Verification items for the finished model (mm, model axes). A direction names the side the tool comes from. Coordinates: 2 decimals unless noted, no trailing zeros. Loops run counter-clockwise (first coordinate to the right, second up) from the corner with the lowest first, then second, coordinate; pieces in that order, holes last.
Q1. Sectioned sample at D-D (z = 3). Enter the section's corners in (x, y).
Q2. Go/stop test with a flat-tipped pin: P1, Ø1, axis at x = -47, z = 6.5, coming from the -Y side. Record where the tip stops, or that it passes through.
Q3. Access from +Z, -Z, +X, -X, +Y, -Y to the whole of each face (thin tool, end or side, straight path). Record for faces 1 (the face through (-30, 2, 30)), 2 (the face through (-30, 0, 21)).
Q4. Material ranges on probe 1 along X at (y, z) = (2.9, 15); probe 2 along Z at (x, y) = (-30, 3.5); probe 3 along X at (y, z) = (-0.25, 16.75), recorded low to high.
Q5. Mould release check, pull along X, two halves, no side actions. Record for faces 3 (the face through (-30, 6, 19)), 4 (the face through (-60, 2, 15)), 5 (the face through (-30, -1, 2)), 6 (the face through (-30, -1, 28)): +X half, -X half, draft (parallel to the pull), parting line (faces both ways), or undercut.
Q6. Sectioned sample at A-A (z = 15). Enter the section's corners in (x, y).
Q7. Sectioned sample at C-C (x = -30). Enter the section's corners in (y, z).
Q8. Sectioned sample at B-B (y = -1). Enter the section's corners in (x, z).
```python
from build123d import *

# Parameters (mm, degrees)
F1_DEPTH       = 6
F2_DEPTH       = 2
F3_D           = 4.2
F3_DEPTH       = 15
F3_CSINK_D     = 8
F3_CSINK_ANGLE = 90
F4_R           = 2


with BuildPart() as f1:
    # F0 (on Front) → F1 (new body)
    with BuildSketch(Plane.XZ):
        Polygon((-60, 0), (0, 0), (0, 30), (-60, 30), (-60, 15), align=None)
        Polygon((-58, 2), (-58, 15), (-58, 28), (-2, 28), (-2, 2), align=None, mode=Mode.SUBTRACT)
        Polygon((-58, 28), (-58, 15), (-58, 2), (-2, 2), (-2, 28), align=None)
    extrude(amount=-F1_DEPTH)

    # F0 (on Front) → F2 (join)
    with BuildSketch(Plane.XZ):
        Polygon((-60, 0), (0, 0), (0, 30), (-60, 30), (-60, 15), align=None)
        Polygon((-58, 2), (-58, 15), (-58, 28), (-2, 28), (-2, 2), align=None, mode=Mode.SUBTRACT)
    extrude(amount=F2_DEPTH)

    # F3
    with Locations(Plane.XZ):
        with Locations((-30, 15)):
            CounterSinkHole(F3_D / 2, F3_CSINK_D / 2, depth=F3_DEPTH, counter_sink_angle=F3_CSINK_ANGLE)

    # F4
    f4_edges = [f1.edges().sort_by_distance(p)[0] for p in [
        (-60, 2, 30),
        (0, 2, 30),
        (0, 2, 0),
        (-60, 2, 0),
    ]]
    fillet(f4_edges, radius=F4_R)


solid = f1.part
```
Geometry check:
1. outline: (-60, -2) - (-58, -2) - (-58, 0) - (-2, 0) - (-2, -2) - (0, -2) - (0, 6) - (-60, 6) - close
2. P1: stops at y = 0
3. face 1: +Z, +X, -X, +Y, -Y
3. face 2: -Y
4. probe 1: x = -60 to -32.1, -27.9 to 0
4. probe 2: z = 0 to 12.9, 17.1 to 30
4. probe 3: x = -60 to -58, -2 to 0
5. face 3: draft
5. face 4: -X half
5. face 5: undercut
5. face 6: undercut
6. outline: (-60, -2) - (-58, -2) - (-58, 0) - (-34, 0) - (-32.1, 1.9) - (-32.1, 6) - (-60, 6) - close; (-27.9, 1.9) - (-26, 0) - (-2, 0) - (-2, -2) - (0, -2) - (0, 6) - (-27.9, 6) - close
7. outline: (-2, 0) - (6, 0) - (6, 12.9) - (1.9, 12.9) - (0, 11) - (0, 2) - (-2, 2) - close; (-2, 28) - (0, 28) - (0, 19) - (1.9, 17.1) - (6, 17.1) - (6, 30) - (-2, 30) - close
8. outline: (-60, 2) arc R2 ccw to (-58, 0) - (-2, 0) arc R2 ccw to (0, 2) - (0, 28) arc R2 ccw to (-2, 30) - (-58, 30) arc R2 ccw to (-60, 28) - close; hole (-58, 2) - (-2, 2) - (-2, 28) - (-58, 28) - close
